```python
from build123d import *

# Parameters (mm, degrees)
BOX004_W     = 45
BOX004_H     = 25
BOX004_DEPTH = 1
BOX001_W     = 115
BOX001_H     = 330
BOX001_DEPTH = 6
BOX005_W     = 45
BOX005_H     = 25
BOX005_DEPTH = 1


with BuildPart() as box004:
    # Box004 → Box004 (new body)
    with BuildSketch(Plane(origin=(35, -25, 2), x_dir=(1, 0, 0), z_dir=(0, 0, 1))):
        with Locations((22.5, 12.5)):
            Rectangle(BOX004_W, BOX004_H)
    extrude(amount=BOX004_DEPTH)


with BuildPart() as box001:
    # Box001 → Box001 (new body)
    with BuildSketch(Plane.XY):
        with Locations((57.5, 165)):
            Rectangle(BOX001_W, BOX001_H)
    extrude(amount=BOX001_DEPTH)


with BuildPart() as fusion003:
    # Box005 → Box005 (new body)
    with BuildSketch(Plane(origin=(35, 330, 2), x_dir=(1, 0, 0), z_dir=(0, 0, 1))):
        with Locations((22.5, 12.5)):
            Rectangle(BOX005_W, BOX005_H)
    extrude(amount=BOX005_DEPTH)

    # Fusion003: union Box004, Box001
    add(box004.part)
    add(box001.part)


solid = fusion003.part
```
Input: part model. Units: mm. Frame: model coordinates. A direction names the side the tool comes from. Coordinates: 2 decimals unless noted, no trailing zeros. Loops run counter-clockwise (first coordinate to the right, second up) from the corner with the lowest first, then second, coordinate; pieces in that order, holes last.
Q1. Line query: line 1 along Z through (x, y) = (68, 339); line 2 along Y through (x, z) = (100, 5.5). Output: solid intervals per line, ascending.
Results are:
line 1: z = 2 to 3
line 2: y = 0 to 330
Q2. Section C-C, the plane x = 94. Return the cut outline in (y, z).
Results are:
outline: (0, 0) - (330, 0) - (330, 6) - (0, 6) - close
Q3. Set-up query: faces 1 (the flat face through (57, 343, 3)), 2 (the flat face through (57, 167, 0)), 3 (the flat face through (57, -12, 3)), 4 (the flat face through (57, 343, 2)), 5 (the flat face through (57, -12, 2)). Return all of +Z, -Z, +X, -X, +Y, -Y with unobstructed straight access to the full face (end or side cutting, diameter ignored); none if empty.
Results are:
face 1: +Z, +X, -X, +Y
face 2: -Z, +X, -X, +Y, -Y
face 3: +Z, +X, -X, -Y
face 4: -Z, +X, -X, +Y
face 5: -Z, +X, -X, -Y
Q4. Section A-A, the plane x = 56. Return the cut outline in (y, z).
Results are:
outline: (-25, 2) - (0, 2) - (0, 0) - (330, 0) - (330, 2) - (355, 2) - (355, 3) - (330, 3) - (330, 6) - (0, 6) - (0, 3) - (-25, 3) - close
Q5. Section B-B, the plane z = 4.55. Return the cut outline in (x, y), and give its area (4 significant figures).
Results are:
outline: (0, 0) - (115, 0) - (115, 330) - (0, 330) - close
area: 37,950 mm2
Q6. Contact query for flat-ended pins moving along their axis: pin 1 (0.5 mm diameter, centred on y = 348.5, z = 2.5, fed in from +X); pin 2 (1.1 mm diameter, centred on y = -11.5, z = 2.5, fed in from -X); pin 3 (7.5 mm diameter, centred on x = 59, y = -12.5, fed in from -Z); pin 4 (3 mm diameter, centred on x = 34, z = 2, fed in from +Y). Output: stop coordinate, or through.
Results are:
pin 1: stops at x = 80
pin 2: stops at x = 35
pin 3: stops at z = 2
pin 4: stops at y = 355
